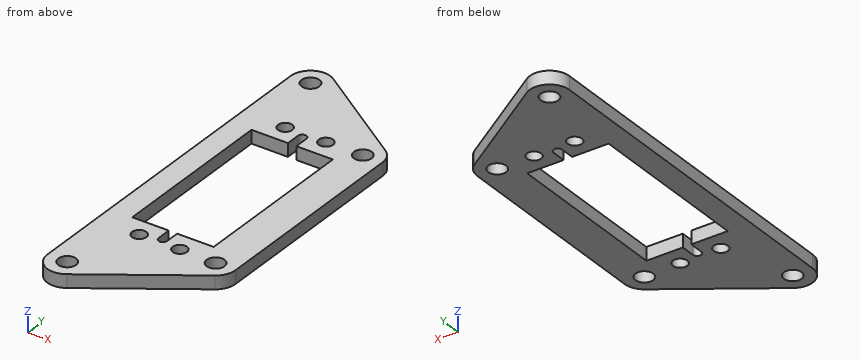
from build123d import *

# Parameters (mm, degrees)
F0_R     = 2.15265
F0_R_2   = 1.7272
F1_DEPTH = 3.175


with BuildPart() as f1:
    # F0 (on Top) → F1 (new body)
    with BuildSketch(Plane.XY):
        with BuildLine():
            Line((18.381172, -25.0825), (18.381172, 25.0825))
            ThreePointArc((18.381172, 25.0825), (17.827276, 27.311637), (16.294431, 29.022261))
            Line((16.294431, 29.022261), (-7.831306, 45.407687))
            ThreePointArc((-7.831306, 45.407687), (-12.736203, 45.676531), (-15.269566, 41.467926))
            Line((-15.269566, 41.467926), (-15.269566, -41.467926))
            ThreePointArc((-15.269566, -41.467926), (-12.736203, -45.676531), (-7.831306, -45.407687))
            Line((-7.831306, -45.407687), (16.294431, -29.022261))
            ThreePointArc((16.294431, -29.022261), (17.827276, -27.311637), (18.381172, -25.0825))
        make_face()
        with Locations((-10.507066, -41.467926)):
            Circle(F0_R, mode=Mode.SUBTRACT)
        with Locations((-4.8895, -24.892)):
            Circle(F0_R_2, mode=Mode.SUBTRACT)
        with BuildLine():
            Line((-1.016, -20.32), (-9.779, -20.32))
            Line((-9.779, -20.32), (-9.779, 20.32))
            Line((-9.779, 20.32), (-1.016, 20.32))
            Line((-1.016, 20.32), (-1.016, 23.749))
            ThreePointArc((-1.016, 23.749), (0, 24.765), (1.016, 23.749))
            Line((1.016, 23.749), (1.016, 20.32))
            Line((1.016, 20.32), (9.779, 20.32))
            Line((9.779, 20.32), (9.779, -20.32))
            Line((9.779, -20.32), (1.016, -20.32))
            Line((1.016, -20.32), (1.016, -23.749))
            ThreePointArc((1.016, -23.749), (0, -24.765), (-1.016, -23.749))
            Line((-1.016, -23.749), (-1.016, -20.32))
        make_face(mode=Mode.SUBTRACT)
        with Locations((4.8895, -24.892)):
            Circle(F0_R_2, mode=Mode.SUBTRACT)
        with Locations((13.618672, -25.0825)):
            Circle(F0_R, mode=Mode.SUBTRACT)
        with Locations((-10.507066, 41.467926)):
            Circle(F0_R, mode=Mode.SUBTRACT)
        with Locations((-4.8895, 24.892)):
            Circle(F0_R_2, mode=Mode.SUBTRACT)
        with Locations((4.8895, 24.892)):
            Circle(F0_R_2, mode=Mode.SUBTRACT)
        with Locations((13.618672, 25.0825)):
            Circle(F0_R, mode=Mode.SUBTRACT)
    extrude(amount=F1_DEPTH)


solid = f1.part
Can you work these out from the model? Positions are in its coordinate system, mm. Coordinates: 2 decimals unless noted, no trailing zeros. Write each loop counter-clockwise with the first axis right and the second up, starting at its lowest first coordinate (ties: lowest second). Pieces come first, ordered by that corner, then holes. Notation, with made-up numbers: (61.5, 84.5) -> (82.5, 84.5) arc R28 cw to (82.5, 119.5) -> close; hole circle Ø11 at (33, 74.25). An arc over 180 degrees is marked (long way). Write item = value, one per line.
(1) If I drill on probe 1 along X at (y, z) = (5, 1.2); probe 2 along Y at (x, z) = (4, 1.75); probe 3 along Y at (x, z) = (-9.5, 2.25), over which ranges is the centre line in solid material (lowest first)?
Verdict:
probe_1 = -15.27 to -9.78, 9.78 to 18.38
probe_2 = -37.37 to -26.37, -23.41 to -20.32, 20.32 to 23.41, 26.37 to 37.37
probe_3 = -46.12 to -43.37, -39.57 to -20.32, 20.32 to 39.57, 43.37 to 46.12
(2) Imagine slicing it at C-C (z = 2.1). State how many separate pieces and enclosed holes the cut face has, and give its area (3 significant figures).
Verdict:
separate_pieces = 1
enclosed_holes = 9
area = 1,680 mm^2
(3) Imagine slicing it at A-A (y = 1.5). Please give me the cut outline in (x, z) (3 decimals).
Verdict:
outline = (-15.27, 0) -> (-9.779, 0) -> (-9.779, 3.175) -> (-15.27, 3.175) -> close; (9.779, 0) -> (18.381, 0) -> (18.381, 3.175) -> (9.779, 3.175) -> close
(4) For pin 1 (3 mm diameter, centred on x = -4.89, y = 24.89, fed in from -Z); pin 2 (1.5 mm diameter, centred on x = -4, z = 1.5, fed in from -Y); pin 3 (1.6 mm diameter, centred on x = 6.5, z = 2, fed in from +Y), each with a flat end and sliding along its axis, tell me the tip position at first contact or that it passes through.
Verdict:
pin_1 = through
pin_2 = -43.31
pin_3 = 36.22
(5) Imagine slicing it at B-B (x = 2). Please give me the cut outline in (y, z) (3 decimals), and give its area (3 significant figures).
Verdict:
outline = (-38.731, 0) -> (-20.32, 0) -> (-20.32, 3.175) -> (-38.731, 3.175) -> close; (20.32, 0) -> (38.731, 0) -> (38.731, 3.175) -> (20.32, 3.175) -> close
area = 117 mm^2
